```python
from build123d import *

# Parameters (mm, degrees)
F0_R      = 55.024553
F1_DEPTH  = 25.4
F2_R      = 38.533102
F2_R_2    = 14.009094
F3_DEPTH  = 25.4
F4_R      = 5.08
F3_FACE_R = 14.009094
F5_DEPTH  = 50.8
F6_R      = 5.08


with BuildPart() as f1:
    # F0 (on Front) → F1 (new body)
    with BuildSketch(Plane.XZ):
        Circle(F0_R)
    extrude(amount=F1_DEPTH)

    # F2 (on face) → F3 (join)
    with BuildSketch(Plane.XZ.offset(25.4)):
        Circle(F2_R)
        Circle(F2_R_2, mode=Mode.SUBTRACT)
    extrude(amount=F3_DEPTH)

    # F4
    f4_edges = [f1.edges().sort_by_distance(p)[0] for p in [
        (-55.024553, -25.4, 0),
        (-38.533102, -50.8, 0),
    ]]
    fillet(f4_edges, radius=F4_R)

    # F3_face (on face) → F5 (join)
    with BuildSketch(Plane.XZ.offset(25.4)):
        Circle(F3_FACE_R)
    extrude(amount=F5_DEPTH)

    # F6
    f6_edges = [f1.edges().sort_by_distance(p)[0] for p in [
        (-14.009094, -76.2, 0),
    ]]
    fillet(f6_edges, radius=F6_R)


solid = f1.part
```
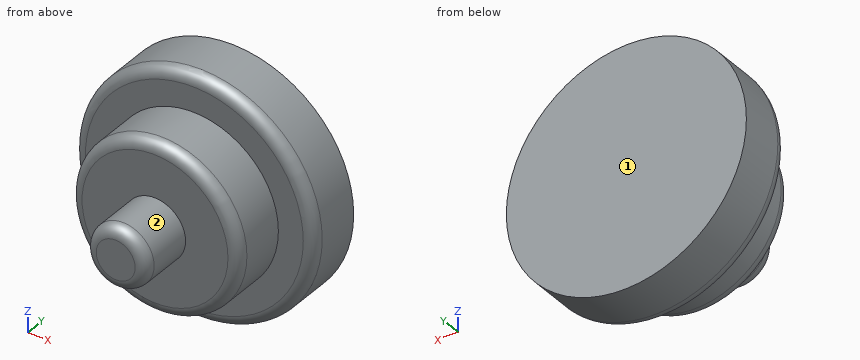
Check sheet for the modelled part. Datum: model origin and axes. Units: mm. Face numbers are marked on the shaded views. A direction names the side the tool comes from. Coordinates: 2 decimals unless noted, no trailing zeros. Write each loop counter-clockwise with the first axis right and the second up, starting at its lowest first coordinate (ties: lowest second). Pieces come first, ordered by that corner, then holes. Notation, with made-up numbers: M 45.5,52.25 L 81.5,52.25 A23 ccw 81.5,79.25 Z; hole C -21,48.25 d4. An arc over 180 degrees is marked long. Write item = value, one per line. Start each with the question number.
1. Tool access check on the marked faces 1 and 2. Record the directions out of +Z, -Z, +X, -X, +Y, -Y that give a thin tool (end or side, any length) a straight path to the whole face; none if there is none.
2. Sectioned sample at A-A (z = 0). Record the cut outline in (x, y), then the cut area to 3 significant figures.
3. Sectioned sample at D-D (y = -34.5). Record the cut outline in (x, z).
4. Sectioned sample at C-C (y = -65). Record the cut outline in (x, z).
5. Go/stop test with flat-tipped pins: pin 1 (3 mm diameter, centred on x = 6.5, z = -31, fed in from -Y); pin 2 (8 mm diameter, centred on y = -31.5, z = -30.5, fed in from -X); pin 3 (12 mm diameter, centred on x = -42.5, z = 33, fed in from -Y). Record where each tip stops, or that it passes through.
6. Sectioned sample at B-B (x = 0). Record the cut outline in (y, z), then the cut area to 3 significant figures.
7. Thickness scan on probe 1 along Z at (x, y) = (0, -13); probe 2 along Y at (x, z) = (-3, -42); probe 3 along Y at (x, z) = (-17.5, -8). Record the ranges inside material, lowest first.
The answers:
q1.face_1 = +Z, -Z, +X, -X, +Y
q1.face_2 = -Y
q2.outline = M -55.02,-20.32 A5.08 ccw -49.94,-25.4 L -38.53,-25.4 L -38.53,-45.72 A5.08 ccw -33.45,-50.8 L -14.01,-50.8 L -14.01,-71.12 A5.08 ccw -8.93,-76.2 L 8.93,-76.2 A5.08 ccw 14.01,-71.12 L 14.01,-50.8 L 33.45,-50.8 A5.08 ccw 38.53,-45.72 L 38.53,-25.4 L 49.94,-25.4 A5.08 ccw 55.02,-20.32 L 55.02,0 L -55.02,0 Z
q2.area = 5,430 mm²
q3.outline = C 0,0 d77.07
q4.outline = C 0,0 d28.02
q5.pin_1 = -50.8
q5.pin_2 = -27.97
q5.pin_3 = -25.4
q6.outline = M -76.2,-8.93 A5.08 ccw -71.12,-14.01 L -50.8,-14.01 L -50.8,-33.45 A5.08 ccw -45.72,-38.53 L -25.4,-38.53 L -25.4,-49.94 A5.08 ccw -20.32,-55.02 L 0,-55.02 L 0,55.02 L -20.32,55.02 A5.08 ccw -25.4,49.94 L -25.4,38.53 L -45.72,38.53 A5.08 ccw -50.8,33.45 L -50.8,14.01 L -71.12,14.01 A5.08 ccw -76.2,8.93 Z
q6.area = 5,430 mm²
q7.probe_1 = -55.02 to 55.02
q7.probe_2 = -25.4 to 0
q7.probe_3 = -50.8 to 0
